Read the model definition and answer for the solid it produces. Units are mm, in the model's axes. A direction names the side the tool comes from. Round coordinates to 2 decimals unless told otherwise and drop trailing zeros. Write each loop counter-clockwise with the first axis right and the second up, starting at its lowest first coordinate (ties: lowest second). Pieces come first, ordered by that corner, then holes. Notation, with made-up numbers: (-39.75, 23.25) -> (-4.75, 23.25) arc R21 cw to (-4.75, 49.25) -> close; hole circle Ø9 at (61.5, 15). An arc over 180 degrees is marked (long way). Return JSON: item names as keys, results as strings.
from build123d import *

# Parameters (mm, degrees)
F1_DEPTH = 25.4
F3_D     = 2.794
F3_DEPTH = 25.4
F3_TIP   = 0.8394022848
F4_D     = 2.794
F4_DEPTH = 25.4
F4_START = 10.1278152
F4_TIP   = 0.8394022848


# Not quite as in the source:
# - ends of sketch curves that miss each other by under 0.0002 mm in the source are joined
# - a feature names something its author has since deleted; it is built from what else it names


with BuildPart() as f1:
    # F0 (on Front) → F1 (new body)
    with BuildSketch(Plane.XZ):
        Polygon((11.0066256276, -6.5430273301), (8.240193387, -9.310965985), (12.5485987193, -9.310965985), (12.5485987193, -1.1086727812), (9.7906497979, 6.8444932552), (24.9488617122, 22.0027051695), (22.8072959293, 24.1442709524), (29.2404852808, 30.5774603039), (22.3196721338, 37.1254323684), (16.0729033236, 30.8786635582), (14.0302290969, 33.0205648235), (13.9806155776, 32.9709513042), (-7.4406042695, 11.5497314571), (-7.4406041338, 11.5466563515), (-7.4413635659, 11.5474157835), (-11.6305711889, -1.2286720797), (-11.6305711889, -9.3063699081), (-7.3613829189, -9.3063699081), (-10.1278151595, -6.5384312532), (-7.4425795762, -3.8636476732), (8.3167760077, -3.8636476732), align=None)
    extrude(amount=F1_DEPTH)

    # F3 (one way)
    with BuildSketch(Plane(origin=(0, 0, 0), x_dir=(0, 1, 0), z_dir=(-1, 0, 0))):
        with Locations((-22.1899207681, 6.5197679214), (-3.1917574815, 6.5197679214)):
            Circle(F3_D / 2)
    extrude(amount=-F3_DEPTH, mode=Mode.SUBTRACT)
    with Locations(Plane(origin=(0, 0, 0), x_dir=(0, 1, 0), z_dir=(-1, 0, 0))):
        with Locations((-22.1899207681, 6.5197679214), (-3.1917574815, 6.5197679214)):
            with Locations((0, 0, -(F3_DEPTH + F3_TIP / 2))):  # 118° drill point
                Cone(0, F3_D / 2, F3_TIP, mode=Mode.SUBTRACT)

    # F4
    # its depths count from where the whole tool has entered the part; down to there all is cleared
    with Locations(Plane.YZ.offset(-F4_START)):
        with Locations((-3.1917574815, -6.5197679214), (-22.1899207681, -6.5197679214)):
            Hole(F4_D / 2, depth=F4_DEPTH)
            with Locations((0, 0, -(F4_DEPTH + F4_TIP / 2))):  # 118° drill point
                Cone(0, F4_D / 2, F4_TIP, mode=Mode.SUBTRACT)


solid = f1.part
Item 1: Straight lines are drawn through the part: L1, parallel to X at y = -12.75, z = 31; L2, parallel to Z at x = 26.5, y = -20.5; L3, parallel to X at y = -20.75, z = -1. For each, find the intervals that lie inside material, in ascending order. Write a range as [from, to].
Worked answers:
{"L1": "x = [12.01, 15.96], [16.19, 28.79]", "L2": "z = [27.84, 33.17]", "L3": "x = [-11.56, 12.51]"}
Item 2: Section A-A (x = 12) is taken. Give the vertices of the cut face in (y, z), then the cut area to 3 significant figures.
Worked answers:
{"outline": "(-25.4, -9.31) -> (0, -9.31) -> (0, 0.47) -> (-25.4, 0.47) -> close; (-25.4, 9.05) -> (0, 9.05) -> (0, 30.99) -> (-25.4, 30.99) -> close; hole circle Ø2.79 at (-22.19, -6.52); hole circle Ø2.79 at (-3.19, -6.52)", "area": "793 mm2"}
Item 3: A tool of negligible diameter and unlimited length cuts with its end or side. For faces 1 (the flat face through (25.979, -12.522, 27.316)), 2 (the flat face through (15.1, -12.5, 31.9)), 3 (the flat face through (9.64, -12.52, -5.18)), from which of +Z, -Z, +X, -X, +Y, -Y can it reach the whole face along a straight path? Write none if from no direction.
Worked answers:
{"face 1": "+X, +Y, -Y", "face 2": "+Z, +Y, -Y", "face 3": "+Y, -Y"}
Item 4: Section B-B (y = -3.75) is taken. State how many separate pieces and enclosed holes the cut face has, then the cut area to 3 significant figures.
Worked answers:
{"separate pieces": "3", "enclosed holes": "0", "area": "788 mm2"}
Item 5: Flat-ended cylindrical pins translate along their axes: pin 1 (1.5 mm diameter, centred on x = -0.5, z = 21, fed in from +Y); pin 2 (3 mm diameter, centred on y = -20, z = 29.5, fed in from +X); pin 3 (3.5 mm diameter, centred on y = -22.19, z = -6.52, fed in from +X); pin 4 (10 mm diameter, centred on y = -8.5, z = 7, fed in from +X). Find the tip coordinate at first contact, or state that the pin passes through.
Worked answers:
{"pin 1": "passes through", "pin 2": "stops at x = 29.24", "pin 3": "stops at x = 12.55", "pin 4": "stops at x = 14.95"}
Item 6: For a pull along Y with two mould halves and no side action, classify faces 4 (the cylindrical face through (11.36, -20.9, -5.98)), 5 (the cylindrical face through (11.365, -1.901, -5.985)), 6 (the flat face through (-11.631, -13, -5)), 7 (the flat face through (9, -25.4, 14)) as released by +Y, released by -Y, zero draft, split by the parting line, or undercut.
Worked answers:
{"face 4": "undercut", "face 5": "undercut", "face 6": "zero draft", "face 7": "released by -Y"}
